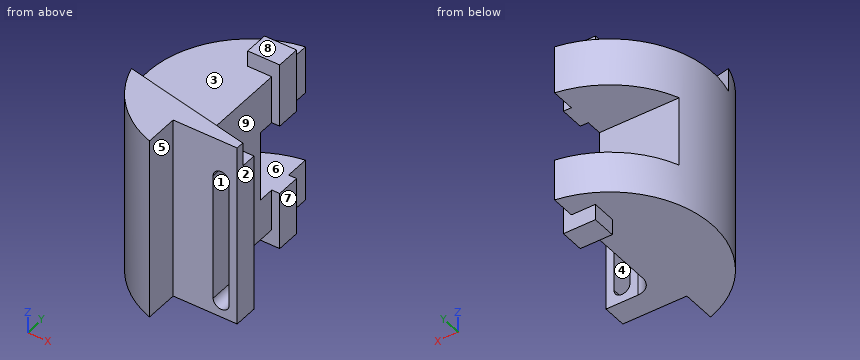
```python
from build123d import *

# Parameters (mm, degrees)
BOSS_EXTRU_1_DEPTH      = 115
ENL_V_START             = -15
ENL_V_MAT_EXTRU_1_DEPTH = 15
BOSS_EXTRU_2_START      = -110
ESQUISSE3_W             = 20
ESQUISSE3_H             = 15
BOSS_EXTRU_2_DEPTH      = 120
ESQUISSE4_W             = 44
ESQUISSE4_H             = 40
ENL_V_MAT_EXTRU_2_DEPTH = 145.095888213
ENL_V_MAT_EXTRU_3_DEPTH = 159.698810645


with BuildPart() as part:
    # Esquisse1 → Boss.-Extru.1 (new body)
    with BuildSketch(Plane.XY):
        with BuildLine():
            Line((-10, 63.467018994), (-10, -15.032981006))
            ThreePointArc((-10, -15.032981006), (-7.071067812, -22.104048818), (0, -25.032981006))
            Line((0, -25.032981006), (20, -25.032981006))
            Line((20, -25.032981006), (20, -40.032981006))
            Line((20, -40.032981006), (-20, -40.032981006))
            Line((-20, -40.032981006), (-20, -61.057861902))
            ThreePointArc((-20, -61.057861902), (-64.043824765, 5.143054489), (-10, 63.467018994))
        make_face()
    extrude(amount=BOSS_EXTRU_1_DEPTH)

    # Esquisse2 → Enlèv. mat.-Extru.1 (cut)
    with BuildSketch(Plane.XY.offset(115).offset(ENL_V_START)):
        with BuildLine():
            Line((20, -35.032981006), (-61.777999904, -17.650530526))
            ThreePointArc((-61.777999904, -17.650530526), (-54.157497427, 34.569176623), (-10, 63.467018994))
            Line((-10, 63.467018994), (-10, -15.032981006))
            ThreePointArc((-10, -15.032981006), (-7.071067812, -22.104048818), (0, -25.032981006))
            Line((0, -25.032981006), (20, -25.032981006))
            Line((20, -25.032981006), (20, -35.032981006))
        make_face()
    extrude(amount=ENL_V_MAT_EXTRU_1_DEPTH, mode=Mode.SUBTRACT)

    # Esquisse3 → Boss.-Extru.2 (add)
    with BuildSketch(Plane.XY.offset(100).offset(BOSS_EXTRU_2_START)):
        with Locations((-15, 40.967018994)):
            Rectangle(ESQUISSE3_W, ESQUISSE3_H)
    extrude(amount=BOSS_EXTRU_2_DEPTH)

    # Esquisse4 → Enlèv. mat.-Extru.2 (cut, through all)
    with BuildSketch(Plane(origin=(-5, 0, 0), x_dir=(0, 0, -1), z_dir=(1, 0, 0))):
        with Locations((-48, 43.467018994)):
            Rectangle(ESQUISSE4_W, ESQUISSE4_H)
    extrude(amount=-ENL_V_MAT_EXTRU_2_DEPTH, mode=Mode.SUBTRACT)

    # Esquisse5 → Enlèv. mat.-Extru.3 (cut, through all)
    with BuildSketch(Plane(origin=(0, -25.032981006, 0), x_dir=(1, 0, 0), z_dir=(0, 1, 0))):
        with BuildLine():
            Line((15, -10), (15, -90))
            ThreePointArc((15, -90), (10, -95), (5, -90))
            Line((5, -90), (5, -10))
            ThreePointArc((5, -10), (10, -5), (15, -10))
        make_face()
    extrude(amount=-ENL_V_MAT_EXTRU_3_DEPTH, mode=Mode.SUBTRACT)


solid = part.part
```
The model under review builds one solid part; all positions refer to its coordinate system, in mm. Face numbers are marked on the shaded views. A direction names the side the tool comes from. Coordinates: 2 decimals unless noted, no trailing zeros. Write each loop counter-clockwise with the first axis right and the second up, starting at its lowest first coordinate (ties: lowest second). Pieces come first, ordered by that corner, then holes.
1) We need section C-C on x = 10. State the section outline as (y, z) points, then the cut area to 3 significant figures.
2) To check wall thickness, follow probe 1 along Z at (x, y) = (-33.5, 24.5); probe 2 along Y at (x, z) = (-0.5, 39.5); probe 3 along Z at (x, y) = (-49.5, 15). State the ranges of each line that lie inside material, in increasing order.
3) We need section B-B on y = 44.5. State the section outline as (x, z) points, then the cut area to 3 significant figures.
4) Machinability: for the marked faces 5, 6, 7, 8 and 9, which of the approach directions +Z, -Z, +X, -X, +Y, -Y give a long, thin tool a straight path to every point of the face, cutting with its end or side? Answer none if there is none.
5) We need section D-D on y = -32.5. State the section outline as (x, z) points, then the cut area to 3 significant figures.
6) We need section A-A on z = 85. State the section outline as (x, y) points, then the cut area to 3 significant figures.
7) Clearance check with flat-ended pins moving along their axes: pin 1 Ø12 at (y, z) = (-35, 46) entering from -X; pin 2 Ø12 at (x, y) = (-43, 49.5) entering from -Z; pin 3 Ø16.5 at (x, y) = (-19, 39) entering from +Z. State where each tip first meets the part, or that it passes through.
8) The part is to be moulded in two halves that separate along X. For the marked faces 1, 2, 3 and 4, say which applies: pulls with the +X half, pulls with the -X half, needs draft (parallel to the pull), parting line crosses it, or undercut.
Answer list:
1. outline: (-40.03, 0) - (-25.03, 0) - (-25.03, 5) - (-40.03, 5) - close; (-40.03, 95) - (-25.03, 95) - (-25.03, 100) - (-32.91, 100) - (-32.91, 115) - (-40.03, 115) - close
1. area: 257 mm2
2. probe 1: z = 0 to 26, 70 to 100
2. probe 2: y = -40.03 to -25.02
2. probe 3: z = 0 to 100
3. outline: (-46.34, 0) - (-25, 0) - (-25, -10) - (-5, -10) - (-5, 26) - (-46.34, 26) - close; (-46.34, 70) - (-5, 70) - (-5, 110) - (-25, 110) - (-25, 100) - (-46.34, 100) - close
3. area: 2,720 mm2
4. face 5: +Z, -Z, +X, -Y
4. face 6: +X, -X, +Y
4. face 7: +Z, -Z, +X, +Y
4. face 8: +Z, +X, -X, +Y
4. face 9: +Z, -Z, +X
5. outline: (-55.42, 0) - (20, 0) - (20, 100) - (8.08, 100) - (8.08, 115) - (-55.42, 115) - close; hole (5, 10) arc R5 ccw to (15, 10) - (15, 90) arc R5 ccw to (5, 90) - close
5. area: 7,620 mm2
6. outline: (-20, -61.06) - (-20, -40.03) - (5, -40.03) - (5, -25.03) - (0, -25.03) arc R10 cw to (-10, -15.03) - (-10, 33.47) - (-5, 33.47) - (-5, 48.47) - (-10, 48.47) - (-10, 63.47) arc R64.25 ccw to start; (15, -40.03) - (20, -40.03) - (20, -25.03) - (15, -25.03) - close
6. area: 5,380 mm2
7. pin 1: stops at x = -57.33
7. pin 2: stops at z = 0
7. pin 3: stops at z = 110
8. face 1: undercut
8. face 2: pulls with the +X half
8. face 3: needs draft
8. face 4: undercut
